```python
from build123d import *

# Parameters (mm, degrees)
F0_W     = 2.54
F0_H     = 12.7
F2_R     = 38.1
F2_R_2   = 33.02
F3_DEPTH = 6.35
F4_R     = 33.02
F4_R_2   = 30.48
F5_DEPTH = 6.35


with BuildPart() as f1:
    # F0 (on Top) → F1 (revolve)
    with BuildSketch(Plane.XY):
        Polygon((-2.54, 12.7), (0, 12.7), (-22.86, 63.5), (-25.4, 63.5), align=None)
        with Locations((-1.27, 6.35)):
            Rectangle(F0_W, F0_H)
    revolve(axis=Axis((7.62, 34.9172540009, 0), (0, 1, 0)))

    # F2 (on face) → F3 (join)
    with BuildSketch(Plane(origin=(0, 63.5, 0), x_dir=(-1, 0, 0), z_dir=(0, 1, 0))):
        with Locations((-7.62, 0)):
            Circle(F2_R)
        Polygon((-41.5798, -1.6002), (-43.18, -1.6002), (-44.7802, -1.6002), (-44.7802, 1.6002), (-43.18, 1.6002), (-41.5798, 1.6002), align=None, mode=Mode.SUBTRACT)
        with Locations((-7.62, 0)):
            Circle(F2_R_2, mode=Mode.SUBTRACT)
        Polygon((27.94, -1.6002), (26.3398, -1.6002), (26.3398, 1.6002), (27.94, 1.6002), (29.5402, 1.6002), (29.5402, -1.6002), align=None, mode=Mode.SUBTRACT)
    extrude(amount=F3_DEPTH)

    # F4 (on face) → F5 (join)
    with BuildSketch(Plane(origin=(0, 63.5, 0), x_dir=(-1, 0, 0), z_dir=(0, 1, 0))):
        with Locations((-7.62, 0)):
            Circle(F4_R)
        with Locations((-7.62, 0)):
            Circle(F4_R_2, mode=Mode.SUBTRACT)
    extrude(amount=F5_DEPTH)


solid = f1.part
```
Part model, mm, in its own coordinate system. A direction names the side the tool comes from. Round coordinates to 2 decimals unless told otherwise and drop trailing zeros. Loops run counter-clockwise (first coordinate to the right, second up) from the corner with the lowest first, then second, coordinate; pieces in that order, holes last.
1. Drill centre lines: line 1 along Z through (x, y) = (7, 7); line 2 along Z through (x, y) = (7.62, 9.5); line 3 along X through (y, z) = (34, -9.5). Where is each one in solid material? Low to high.
Solutions:
line 1: z = -10.14 to -7.59, 7.59 to 10.14
line 2: z = -10.16 to -7.62, 7.62 to 10.16
line 3: x = -9.69 to -6.72, 21.96 to 24.93
2. Slice it at C-C (y = 11). Give the cut face in (x, z).
Solutions:
outline: circle Ø20.32 at (7.62, 0); hole circle Ø15.24 at (7.62, 0)
3. Slice it at D-D (y = 41.5). Give the cut face in (x, z), and give its area (3 significant figures).
Solutions:
outline: circle Ø46.24 at (7.62, 0); hole circle Ø41.16 at (7.62, 0)
area: 349 mm2
4. Flat gauge pins, fed straight in: pin 1 (2.5 mm diameter, centred on y = 65.5, z = 0.5, fed in from +X); pin 2 (2.5 mm diameter, centred on x = 42.5, y = 66.5, fed in from -Z); pin 3 (3.5 mm diameter, centred on x = -28, y = 65.5, fed in from -Z); pin 4 (1 mm diameter, centred on x = 17, z = 13.5, fed in from +Y). Where does each tip first touch, or does it go through?
Solutions:
pin 1: stops at x = 45.72
pin 2: stops at z = -17.91
pin 3: stops at z = -17.45
pin 4: stops at y = 33.41
5. Slice it at B-B (x = 7.62). Give the cut face in (y, z).
Solutions:
outline: (0, -10.16) - (12.7, -10.16) - (63.5, -33.02) - (63.5, -38.1) - (69.85, -38.1) - (69.85, -30.48) - (63.5, -30.48) - (12.7, -7.62) - (0, -7.62) - close; (0, 7.62) - (12.7, 7.62) - (63.5, 30.48) - (69.85, 30.48) - (69.85, 38.1) - (63.5, 38.1) - (63.5, 33.02) - (12.7, 10.16) - (0, 10.16) - close
6. Two-plate mould, pull along X, no slides. Class faces 5 (the face through (17.77, 6.44, 0.45)), 6 (the face through (41.58, 67, 0)), 7 (the face through (33.2, 69.85, 17.1)): pulls with the +X half, pulls with the -X half, needs draft (parallel to the pull), parting line crosses it, or undercut.
Solutions:
face 5: parting line crosses it
face 6: undercut
face 7: needs draft
7. 3-axis set-ups, long thin cutter, end or side, ignore diameter. For faces 1 (the face through (14.227, 66.631, -29.755)), 2 (the face through (39, 63.5, -11)), 3 (the face through (-28, 67, 1.6)), 4 (the face through (6, 0, 8)): which of +Z, -Z, +X, -X, +Y, -Y reach the whole face in a straight line?
Solutions:
face 1: +Y
face 2: -Y
face 3: +Y, -Y
face 4: +Z, -Z, +X, -X, -Y
8. Slice it at A-A (z = 0). Give the cut face in (x, y).
Solutions:
outline: (-30.48, 63.5) - (-29.54, 63.5) - (-29.54, 69.85) - (-30.48, 69.85) - close; (-26.34, 63.5) - (-25.4, 63.5) - (-2.54, 12.7) - (-2.54, 0) - (0, 0) - (0, 12.7) - (-22.86, 63.5) - (-22.86, 69.85) - (-26.34, 69.85) - close; (15.24, 0) - (17.78, 0) - (17.78, 12.7) - (40.64, 63.5) - (41.58, 63.5) - (41.58, 69.85) - (38.1, 69.85) - (38.1, 63.5) - (15.24, 12.7) - close; (44.78, 63.5) - (45.72, 63.5) - (45.72, 69.85) - (44.78, 69.85) - close
